Geometry: final body of the model. Coordinates: model frame, mm. A direction names the side the tool comes from. Round coordinates to 2 decimals unless told otherwise and drop trailing zeros. Loops run counter-clockwise (first coordinate to the right, second up) from the corner with the lowest first, then second, coordinate; pieces in that order, holes last. Notation, with made-up numbers: M -38,23 L 12,23 A34 ccw 12,60 Z; hole C 26.25,4.5 d2. An arc over 180 degrees is marked long. Return JSON: item names as keys, results as strings.
from build123d import *

# Parameters (mm, degrees)
SKETCH_R             = 10
PAD_DEPTH            = 26
SKETCH006_R          = 1.2
POCKET_DEPTH         = 10.001
POCKET_DEPTH_BACK    = 10.001
BODY_PLACEMENT_ANGLE = 180


with BuildPart() as part:
    # Sketch → Pad (new body)
    with BuildSketch(Plane.XY):
        Circle(SKETCH_R)
        with BuildLine():
            ThreePointArc((-1.265543, 1.6), (0, -2.04), (1.265543, 1.6))
            Line((-1.265543, 1.6), (1.265543, 1.6))
        make_face(mode=Mode.SUBTRACT)
    extrude(amount=PAD_DEPTH)

    # Sketch001 → Groove (revolve, cut)
    with BuildSketch(Plane.XZ):
        Polygon((10, 25.33014), (3, 20.5), (3, 5.5), (10, 4), align=None)
    revolve(axis=Axis((0, 0, 0), (0, 0, 1)), mode=Mode.SUBTRACT)

    # Sketch006 → Pocket (cut, two sides)
    with BuildSketch(Plane.XZ) as pocket_sk:
        with Locations((0, 13)):
            Circle(SKETCH006_R)
    extrude(amount=-POCKET_DEPTH, mode=Mode.SUBTRACT)
    extrude(pocket_sk.sketch, amount=POCKET_DEPTH_BACK, mode=Mode.SUBTRACT)


with BuildPart() as part_1:
    # Body placement: moved
    add(part.part.moved(Location((0, 0, -5))).rotate(Axis((0, 0, -5), (0, 1, 0)), BODY_PLACEMENT_ANGLE))


solid = part_1.part
Q1. Section query C-C (z = -22). Output: boundary loops of the cut face in (x, y).
Determined:
{"outline": "C 0,0 d6; hole M -1.27,1.6 A2.04 ccw long 1.27,1.6 Z"}
Q2. Section query B-B (z = -18). Output: boundary loops of the cut face in (x, y).
Determined:
{"outline": "M -1.27,1.6 L -1.2,1.6 L -1.2,2.75 A3 ccw -1.2,-2.75 L -1.2,-1.65 A2.04 cw Z; M 1.2,-2.75 A3 ccw 1.2,2.75 L 1.2,1.6 L 1.27,1.6 A2.04 cw 1.2,-1.65 Z"}
Q3. Pull-direction query (Y, two-part tool) for faces 1 (the cylindrical face through (2.17, -9.76, -6.97)), 2 (the flat face through (2.4, 0.1, -31)), 3 (the flat face through (0, 1.6, -15)); classes: pulls with the +Y half, pulls with the -Y half, needs draft (parallel to the pull), parting line crosses it, or undercut.
Determined:
{"face 1": "parting line crosses it", "face 2": "needs draft", "face 3": "undercut"}
Q4. Section query D-D (z = -9.5). Output: boundary loops of the cut face in (x, y), plus the area to 3 significant figures.
Determined:
{"outline": "C 0,0 d15.33; hole M -1.27,1.6 A2.04 ccw long 1.27,1.6 Z", "area": "172 mm^2"}
Q5. Pin query (flat end, axial travel): pin 1 (1.4 mm diameter, centred on x = 0, z = -18, fed in from -Y); pin 2 (4 mm diameter, centred on x = -0.5, z = -17.5, fed in from +Y); pin 3 (10 mm diameter, centred on y = -1, z = -21.5, fed in from -X); pin 4 (8 mm diameter, centred on y = -2, z = -15.5, fed in from -X). Return the tip coordinate at first contact, or that it passes through.
Determined:
{"pin 1": "passes through", "pin 2": "stops at y = 3", "pin 3": "stops at x = -4.39", "pin 4": "stops at x = -3"}
Q6. Reachability of faces 4 (the cylindrical face through (-1.11, 2.29, -17.54)), 5 (the conical face through (0.724, -3.26, -25.735)) from +Z, -Z, +X, -X, +Y, -Y: full face, straight path, thin tool, end or side. Return the list, or none.
Determined:
{"face 4": "+Y, -Y", "face 5": "none"}
Q7. Section query A-A (x = 0). Output: boundary loops of the cut face in (y, z), plus the area to 3 significant figures.
Determined:
{"outline": "M -10,-31 L -2.04,-31 L -2.04,-19.2 L -3,-19.2 L -3,-25.5 L -10,-30.33 Z; M -10,-9 L -3,-10.5 L -3,-16.8 L -2.04,-16.8 L -2.04,-5 L -10,-5 Z; M 1.6,-31 L 10,-31 L 10,-30.33 L 3,-25.5 L 3,-19.2 L 1.6,-19.2 Z; M 1.6,-16.8 L 3,-16.8 L 3,-10.5 L 10,-9 L 10,-5 L 1.6,-5 Z", "area": "165 mm^2"}
Q8. Material intervals for L1, parallel to Z at x = 0, y = 2.1; L2, parallel to Z at x = -3.25, y = 2.25; L3, parallel to X at y = 1, z = -11, sorted ascending.
Determined:
{"L1": "z = -31 to -19.2, -16.8 to -5", "L2": "z = -31 to -26.16, -10.3 to -5", "L3": "x = -2.83 to -1.78, 1.78 to 2.83"}
